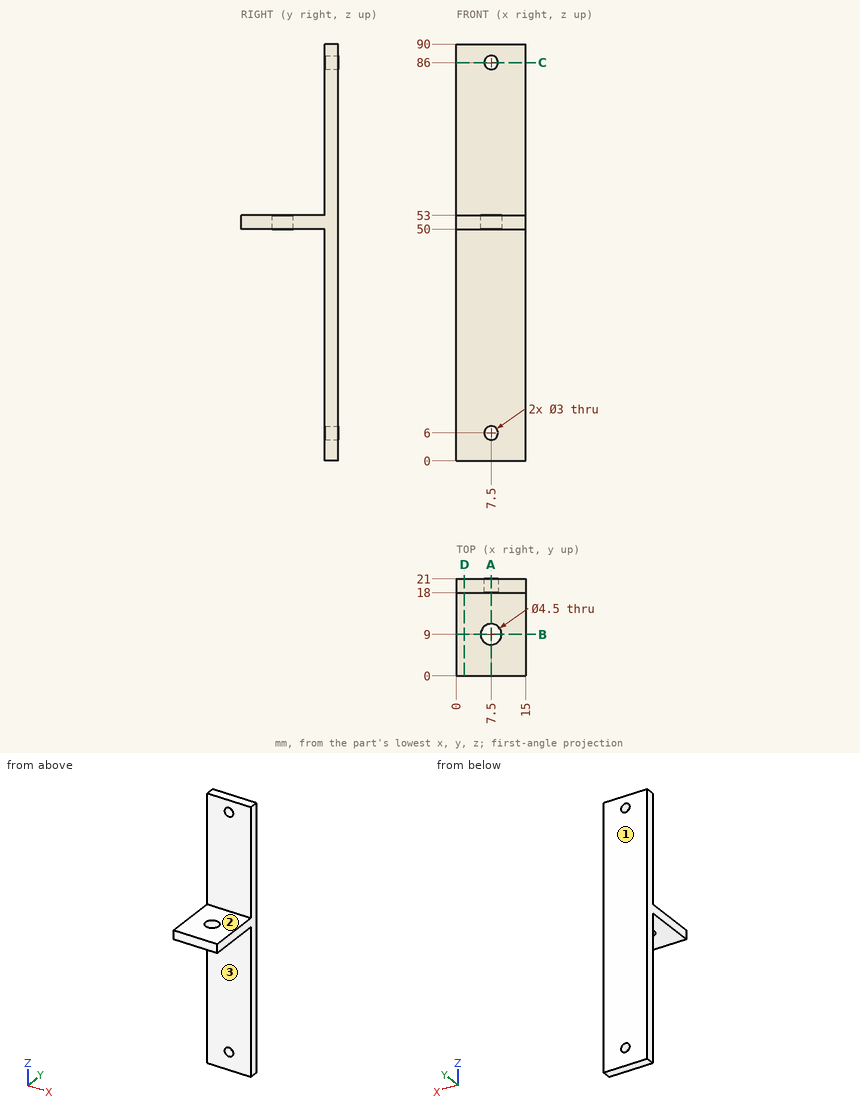
Here's the drawing with two shaded views (mm, measured from the low corner). I have some questions. A direction names the side the tool comes from. Give positions to 0.01 mm unless a question says otherwise; leave off trailing zeros. Loops run counter-clockwise (first coordinate to the right, second up) from the corner with the lowest first, then second, coordinate; pieces in that order, holes last. Notation, with made-up numbers: (45.25, -32.75) -> (87.25, -32.75) arc R33 cw to (87.25, 5.25) -> close; hole circle Ø8 at (46.25, -32). An arc over 180 degrees is marked (long way). Answer as a JSON object with one key per item and string values. Group by question number.
Item 1: Imagine slicing it at B-B on y = 9. Write out the boundary of the cut face in (x, z), then the cut area to 3 significant figures.
Item 2: Imagine slicing it at A-A on x = 7.5. Write out the boundary of the cut face in (y, z), then the cut area to 4 significant figures.
Item 3: Imagine slicing it at C-C on z = 86. Write out the boundary of the cut face in (x, y).
Item 4: I need wall thicknesses on L1, parallel to Z at x = 7.5, y = 19; L2, parallel to Y at x = 7.5, z = 50.95; L3, parallel to X at y = 19.2, z = 86. Which ranges of each line are inside material? Lowest first, please.
Item 5: On a 3-axis mill with a long thin cutter (end or side, diameter ignored), from which of +Z, -Z, +X, -X, +Y, -Y can I reach the whole of each face in a straight line? I mean the marked faces 1, 2 and 3. Say none if no direction works.
Item 6: Imagine slicing it at D-D on x = 1.75. Write out the boundary of the cut face in (y, z), then the cut area to 3 significant figures.
Item 7: Will these pins go through, and if not, where does the flat tip stop? pin 1 (4.5 mm diameter, centred on x = 5.5, y = 5, fed in from -Z); pin 2 (6 mm diameter, centred on x = 13, z = 14, fed in from -Y); pin 3 (8 mm diameter, centred on x = 7, y = 10, fed in from +Z).
Answer list:
{
 "1": {"outline": "(0, 50) -> (5.25, 50) -> (5.25, 53) -> (0, 53) -> close; (9.75, 50) -> (15, 50) -> (15, 53) -> (9.75, 53) -> close", "area": "31.5 mm2"},
 "2": {"outline": "(0, 50) -> (6.75, 50) -> (6.75, 53) -> (0, 53) -> close; (11.25, 50) -> (18, 50) -> (18, 7.5) -> (21, 7.5) -> (21, 84.5) -> (18, 84.5) -> (18, 53) -> (11.25, 53) -> close; (18, 0) -> (21, 0) -> (21, 4.5) -> (18, 4.5) -> close; (18, 87.5) -> (21, 87.5) -> (21, 90) -> (18, 90) -> close", "area": "292.5 mm2"},
 "3": {"outline": "(0, 18) -> (6, 18) -> (6, 21) -> (0, 21) -> close; (9, 18) -> (15, 18) -> (15, 21) -> (9, 21) -> close"},
 "4": {"L1": "z = 0 to 4.5, 7.5 to 84.5, 87.5 to 90", "L2": "y = 0 to 6.75, 11.25 to 21", "L3": "x = 0 to 6, 9 to 15"},
 "5": {"face 1": "+Z, -Z, +X, -X, +Y", "face 2": "+Z, +X, -X, -Y", "face 3": "-Z, +X, -X, -Y"},
 "6": {"outline": "(0, 50) -> (18, 50) -> (18, 0) -> (21, 0) -> (21, 90) -> (18, 90) -> (18, 53) -> (0, 53) -> close", "area": "324 mm2"},
 "7": {"pin 1": "stops at z = 50", "pin 2": "stops at y = 18", "pin 3": "stops at z = 53"}
}
